Autodesk Inventor part; units mm, degrees
ref_plane "YZ Plane" through (0, 0, 0) normal (1, 0, 0) x (0, 1, 0)
ref_plane "XZ Plane" through (0, 0, 0) normal (0, 1, 0) x (-1, 0, 0)
ref_plane "XY Plane" through (0, 0, 0) normal (0, 0, 1) x (1, 0, 0)
sketch "Sketch1" plane through (0, 0, 0) normal (0, 1, 0) x (-1, 0, 0)
  line L0 (-22.5, 32.5) -> (22.5, 32.5) construction
  line L1 (22.5, 32.5) -> (22.5, -32.5) construction
  line L2 (22.5, -32.5) -> (-22.5, -32.5) construction
  line L3 (-22.5, -32.5) -> (-22.5, 32.5) construction
  line L4 (-22.5, 32.5) -> (22.5, -32.5) construction
  line L5 (22.5, 32.5) -> (-22.5, -32.5) construction
  circle A0 centre (22.5, 32.5) radius 1.5
  circle A1 centre (22.5, -32.5) radius 1.5
  circle A2 centre (-22.5, -32.5) radius 1.5
  circle A3 centre (-22.5, 32.5) radius 1.5
  line L6 (27.5, 30) -> (-27.5, 30)
  line L7 (-27.5, 30) -> (-27.5, 37.5)
  line L8 (-27.5, 37.5) -> (27.5, 37.5)
  line L9 (27.5, 37.5) -> (27.5, 30)
  line L10 (27.5, -30) -> (27.5, -37.5)
  line L11 (27.5, -37.5) -> (-27.5, -37.5)
  line L12 (-27.5, -37.5) -> (-27.5, -30)
  line L13 (-27.5, -30) -> (27.5, -30)
  circle A4 centre (22.5, 32.5) radius 5
  circle A5 centre (22.5, -32.5) radius 5
  circle A6 centre (-22.5, -32.5) radius 5
  circle A7 centre (-22.5, 32.5) radius 5
  line L14 (-27.5, 37.5) -> (27.5, 37.5)
  line L15 (27.5, 37.5) -> (27.5, -37.5)
  line L16 (27.5, -37.5) -> (-27.5, -37.5)
  line L17 (-27.5, -37.5) -> (-27.5, 37.5)
  line L18 (-27.5, 37.5) -> (27.5, -37.5) construction
  line L19 (27.5, 37.5) -> (-27.5, -37.5) construction
  line L20 (-32.5, 42.5) -> (32.5, 42.5)
  line L21 (32.5, 42.5) -> (32.5, -42.5)
  line L22 (32.5, -42.5) -> (-32.5, -42.5)
  line L23 (-32.5, -42.5) -> (-32.5, 42.5)
  line L24 (-32.5, 42.5) -> (32.5, -42.5) construction
  line L25 (32.5, 42.5) -> (-32.5, -42.5) construction
  line L26 (32.5, 42.5) -> (-14.872, 42.5)
  line L27 (0, 0) -> (0, -184) construction
  line L28 (-21, -47.5) -> (21, -47.5)
  line L29 (21, -47.5) -> (21, -89.5)
  line L30 (21, -89.5) -> (-21, -89.5)
  line L31 (-21, -89.5) -> (-21, -47.5)
  line L32 (-21, -47.5) -> (21, -89.5) construction
  line L33 (21, -47.5) -> (-21, -89.5) construction
  line L34 (32.5, -42.5) -> (32.5, -94.5)
  line L35 (32.5, -94.5) -> (-32.5, -94.5)
  line L36 (-32.5, -94.5) -> (-32.5, -42.5)
  line L37 (22.5, 27.5) -> (27.5, 27.5)
  line L38 (22.5, -27.5) -> (27.5, -27.5)
  line L39 (-22.5, -27.5) -> (-27.5, -27.5)
  line L40 (-22.5, 27.5) -> (-27.5, 27.5)
  line L41 (0, 0) -> (0, 113) construction
  line L42 (32.5, 42.5) -> (32.5, 97.5)
  line L43 (32.5, 97.5) -> (-32.5, 97.5)
  line L44 (-32.5, 97.5) -> (-32.5, 42.5)
  line L45 (29.5, 42.5) -> (29.5, 97.5)
  line L46 (-29.5, 97.5) -> (-29.5, 42.5)
  line L47 (32.5, 42.5) -> (36.5, 42.5)
  line L48 (36.5, 42.5) -> (36.5, 112.5)
  line L49 (36.5, 112.5) -> (-36.5, 112.5)
  line L50 (-36.5, 112.5) -> (-36.5, 42.5)
  line L51 (-36.5, 42.5) -> (-32.5, 42.5)
  line L52 (-27.5, 37.5) -> (-36.5, 37.5)
  line L53 (-36.5, 37.5) -> (-36.5, 42.5)
  line L54 (-27.5, -27.5) -> (-26.5, -27.5)
  line L55 (-26.5, -27.5) -> (-26.5, 27.5)
  line L56 (0, 112.5) -> (0, 97.5)
  line L57 (-25.05, 112.5) -> (25.05, 112.5)
  line L58 (25.05, 112.5) -> (25.05, 97.5)
  line L59 (25.05, 97.5) -> (-25.05, 97.5)
  line L60 (-25.05, 97.5) -> (-25.05, 112.5)
  line L61 (-25.05, 112.5) -> (25.05, 97.5) construction
  line L62 (25.05, 112.5) -> (-25.05, 97.5) construction
  line L63 (25.05, 109.5) -> (-25.05, 109.5)
  line L64 (36.5, 112.5) -> (-36.5, 112.5)
  line L65 (-36.5, 112.5) -> (-36.5, 116.5)
  line L66 (-36.5, 116.5) -> (36.5, 116.5)
  line L67 (36.5, 116.5) -> (36.5, 112.5)
  line L68 (36.5, 42.5) -> (36.5, 37.5)
  line L69 (36.5, 37.5) -> (32.5, 37.5)
  point P0 (0, -68.5)
  point P1 (18.1699, 30)
  point P2 (18.1699, -30)
  point P3 (-18.1699, -30)
  point P4 (-18.1699, 30)
  point P5 (-32.5, 70)
  point P6 (32.5, 0)
  point P7 (-32.5, 37.5)
  point P8 (0, 105)
  point P9 (-25.05, 97.5)
  dimension "d8" = 10
  dimension "d9" = 10
  dimension "d10" = 10
  dimension "d11" = 10
  dimension "d0" = 45
  dimension "d1" = 65
  dimension "d2" = 3
  dimension "d3" = 3
  dimension "d4" = 3
  dimension "d5" = 3
  dimension "d6" = 2.5
  dimension "d7" = 2.5
  dimension "d12" = 5
  dimension "d13" = 5
  dimension "d17" = 42
  dimension "d18" = 42
  dimension "d19" = 5
  dimension "d20" = 5
  dimension "d38" = 55
  dimension "d39" = 3
  dimension "d40" = 3
  dimension "d41" = 4
  dimension "d42" = 4
  dimension "d43" = 15
  dimension "d57" = 1
  dimension "d72" = 50.1
  dimension "d84" = 7
  dimension "d85" = 3
extrude "Extrusion1" add sketch "Sketch1" along normal blind 6 contours L15 L37 A4 L6 | L6 A4 L9 | L23 L20 L21 L22 | L52 L53 L51 L23 | A4 L6 | L6 A4 | A4 L8 L9 | L6 A7 L8 A4 | L15 L13 A5 L38 | A7 L6 | L6 A7 | A7 L7 L8 | L10 A5 L13 | A5 L13 | A7 L40 L17 L6 | L6 L7 A7 | A5 L13 | L10 L11 A5 | A5 L11 A6 L13 | A6 L13 | L13 A6 | L39 A6 L13 L17 | L22 L34 L35 L36 | L44 L43 L46 L20 | L51 L50 L49 L60 L43 L44 | L11 L12 A6 | A6 L12 L13 | L21 L47 L68 L69 | L65 L66 L67 L49 | L20 L45 L43 L42 | L42 L43 L58 L49 L48 L47 | L49 L56 L63 L60 | L49 L58 L63 L56 | L28 L29 L30 L31
sketch "Sketch3" plane through (0, 6, 0) normal (0, 1, 0) x (1, 0, 0)
  line L0 (-29.5, -97.5) -> (-29.5, -42.5)
  line L1 (-29.5, -42.5) -> (29.5, -42.5)
  circle A0 centre (-22.5, -32.5) radius 1.5
  circle A1 centre (22.5, 32.5) radius 1.5
  circle A2 centre (22.5, -32.5) radius 1.5
  circle A3 centre (-22.5, 32.5) radius 1.5
  arc A4 (-18.1699, -30) -> (-22.5, -27.5) centre (-22.5, -32.5) ccw
  line L2 (-22.5, -27.5) -> (-27.5, -27.5)
  line L3 (-27.5, -27.5) -> (-27.5, 27.5)
  line L4 (-27.5, 27.5) -> (-22.5, 27.5)
  arc A5 (-22.5, 27.5) -> (-18.1699, 30) centre (-22.5, 32.5) ccw
  line L5 (-18.1699, 30) -> (18.1699, 30)
  arc A6 (18.1699, 30) -> (22.5, 27.5) centre (22.5, 32.5) ccw
  line L6 (22.5, 27.5) -> (27.5, 27.5)
  line L7 (27.5, 27.5) -> (27.5, -27.5)
  line L8 (27.5, -27.5) -> (22.5, -27.5)
  arc A7 (22.5, -27.5) -> (18.1699, -30) centre (22.5, -32.5) ccw
  line L9 (18.1699, -30) -> (-18.1699, -30)
  line L10 (32.5, -37.5) -> (32.5, 94.5)
  line L11 (32.5, 94.5) -> (-32.5, 94.5)
  line L12 (-32.5, 94.5) -> (-32.5, -37.5)
  line L13 (-29.5, -97.5) -> (-32.5, -97.5)
  line L14 (-29.5, -97.5) -> (-29.5, -42.5)
  line L15 (-29.5, -42.5) -> (-32.5, -42.5)
  line L16 (-32.5, -42.5) -> (-32.5, -97.5)
  line L17 (29.5, -97.5) -> (32.5, -97.5)
  line L18 (32.5, -97.5) -> (32.5, -42.5)
  line L19 (32.5, -42.5) -> (29.5, -42.5)
  line L20 (-32.5, 0) -> (-27.5, 0)
  line L21 (-27.5, 27.5) -> (-27.5, 94.5)
  line L22 (27.5, 27.5) -> (27.5, 94.5)
  line L23 (32.5, 94.5) -> (-32.5, 94.5)
  line L24 (36.5, -37.5) -> (32.5, -37.5)
  line L25 (27.5, -27.5) -> (27.5, -42.5)
  line L26 (32.5, -31.5) -> (27.5, -31.5)
  line L27 (32.5, -2.5) -> (27.5, -2.5)
  line L28 (27.5, -31.5) -> (27.5, -2.5)
  line L29 (27.5, -17) -> (32.5, -17) construction
  line L30 (-25.05, -97.5) -> (-29.5, -97.5)
  line L31 (-36.5, -116.5) -> (36.5, -116.5)
  line L32 (36.5, -116.5) -> (36.5, -37.5)
  line L33 (-32.5, -37.5) -> (-36.5, -37.5)
  line L34 (-36.5, -37.5) -> (-36.5, -116.5)
  line L35 (29.5, -42.5) -> (29.5, -97.5)
  line L36 (29.5, -97.5) -> (25.05, -97.5)
  line L37 (25.05, -97.5) -> (25.05, -109.5)
  line L38 (25.05, -109.5) -> (-25.05, -109.5)
  line L39 (-25.05, -109.5) -> (-25.05, -97.5)
  line L40 (-27.5, -27.5) -> (-27.5, -42.5)
  line L41 (27.5, 89.5) -> (-27.5, 89.5)
  point P0 (0, 0)
  point P1 (27.5, 0)
  point P2 (30, -2.5)
  point P3 (30, -31.5)
  point P4 (-32.5, -42.5)
  dimension "d44" = 3
  dimension "d45" = 3
  dimension "d48" = 29
  dimension "d49" = 1
  dimension "d107" = 5
extrude "Extrusion3" add sketch "Sketch3" along normal blind 45 contours L13 L16 L15 L0 | L30 L39 L38 L37 L36 L17 L18 L19 L1 L25 L26 L10 L24 L32 L31 L34 L33 L12 L20 L3 L40 L15 L16 L13 | L19 L18 L17 L35 | L25 L7 L27 L10 L26 | L20 L12 L11 L21 L3 | L7 L22 L11 L10 L27 | L21 L11 L22 L41
sketch "Sketch7" plane through (25.05, 0, 109.5) normal (0, 0, -1) x (-1, 0, 0)
  line L0 (4.05, 6) -> (46.05, 6)
  line L1 (0, 0) -> (50.1, 0)
  line L2 (50.1, 0) -> (50.1, 51)
  line L3 (0, 0) -> (0, 51)
  line L4 (25.05, 51) -> (25.05, 0) construction
  line L5 (5.05, 46) -> (45.05, 46)
  line L6 (45.05, 46) -> (45.05, 6)
  line L7 (45.05, 6) -> (5.05, 6)
  line L8 (5.05, 6) -> (5.05, 46)
  line L9 (5.05, 46) -> (45.05, 6) construction
  line L10 (45.05, 46) -> (5.05, 6) construction
  circle A0 centre (45.05, 6) radius 2
  circle A1 centre (45.05, 46) radius 2
  circle A2 centre (5.05, 46) radius 2
  circle A3 centre (5.05, 6) radius 2
  circle A4 centre (25.05, 26) radius 25
  line L11 (0, 51) -> (50.1, 51)
  dimension "d74" = 40
  dimension "d75" = 40
  dimension "d77" = 4
  dimension "d78" = 4
  dimension "d79" = 4
  dimension "d80" = 4
  dimension "d81" = 50
  dimension "d86" = 6
extrude "Extrusion9" cut sketch "Sketch7" against normal blind 45 contours A4 L8 L5 L6 L0 | L0 A4 | A4 L8 | L6 A4 | A4 L5
extrude "Extrusion10" cut sketch "Sketch7" against normal blind 5 contours L8 A3 L0 | L0 A3 L8 | A0 L6 L0 | L0 L6 A0 | A2 L5 L8 | L8 L5 A2 | A1 L5 L6 | L6 L5 A1
sketch "Sketch8" plane through (0, 51, 0) normal (0, 1, 0) x (1, 0, 0)
  line L0 (32.5, 94.5) -> (-32.5, 94.5)
  line L1 (-32.5, 94.5) -> (-32.5, -37.5)
  line L2 (-36.5, -116.5) -> (0, -116.5)
  line L3 (36.5, -116.5) -> (36.5, -37.5)
  line L4 (36.5, -37.5) -> (32.5, -37.5)
  line L5 (32.5, -37.5) -> (32.5, 94.5)
  line L6 (-36.5, -42.5) -> (36.5, -42.5)
  line L7 (-32.5, -37.5) -> (-36.5, -37.5)
  line L8 (-36.5, -37.5) -> (-36.5, -116.5)
  line L9 (0, -109.5) -> (0, -116.5)
  line L10 (0, -116.5) -> (36.5, -116.5)
  line L11 (27.5, -42.5) -> (29.5, -42.5)
  line L12 (29.5, -42.5) -> (29.5, -97.5)
  line L13 (29.5, -97.5) -> (25.05, -97.5)
  line L14 (25.05, -97.5) -> (25.05, -109.5)
  line L15 (25.05, -109.5) -> (0, -109.5)
  line L16 (0, -109.5) -> (-25.05, -109.5)
  line L17 (-25.05, -109.5) -> (-25.05, -97.5)
  line L18 (-25.05, -97.5) -> (-29.5, -97.5)
  line L19 (-29.5, -97.5) -> (-29.5, -42.5)
  line L20 (27.5, 89.5) -> (27.5, -42.5)
  line L21 (-29.5, -42.5) -> (-27.5, -42.5)
  line L22 (-27.5, -42.5) -> (-27.5, 89.5)
  line L23 (-27.5, 89.5) -> (27.5, 89.5)
  point P0 (0, 0)
extrude "Extrusion11" add sketch "Sketch8" along normal blind 4 contours L5 L4 L3 L6 L20 L23 L22 L8 L7 L1 L0 | L3 L10 L9 L15 L14 L13 L12 L6 | L6 L19 L18 L17 L16 L9 L2 L8
properties part number "New_base_v2"
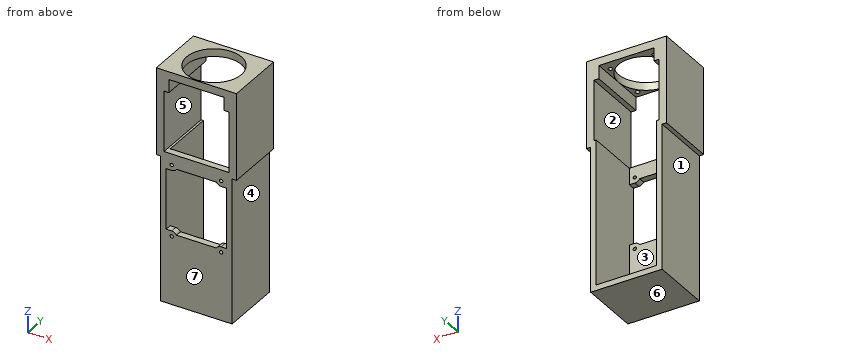
Work out the finished part from the listing and answer in its coordinate system (mm). Face numbers are marked on the shaded views. A direction names the side the tool comes from. Round coordinates to 2 decimals unless told otherwise and drop trailing zeros. Write each loop counter-clockwise with the first axis right and the second up, starting at its lowest first coordinate (ties: lowest second). Pieces come first, ordered by that corner, then holes.
1) A cutting plane is placed at B-B on x = 0. Determine the outline of the cut face in (y, z).
2) Consider probe 1 along X at (y, z) = (35.5, -79.5); probe 2 along Z at (x, y) = (-22.5, 2.6); probe 3 along X at (y, z) = (26, 111). Determine where each line is inside the solid, lowest interval first.
3) Flat-ended cylindrical pins translate along their axes: P1, Ø5, axis at y = 14.5, z = 32, coming from the -X side; P2, Ø16.5, axis at x = -7.5, y = 39, coming from the +Z side; P3, Ø4.5, axis at x = 35, y = 39, coming from the -Z side. Find the tip coordinate at first contact, or state that the pin passes through.
4) Which of the six approach directions +Z, -Z, +X, -X, +Y, -Y give full straight-line access (tool end or side, diameter ignored) to the marked faces 1, 2, 3 and 4?
5) Determine the mould class of the marked faces 5, 6 and 7 for opening direction Z: pulls with the +Z half, pulls with the -Z half, needs draft (parallel to the pull), parting line crosses it, or undercut.
6) A cutting plane is placed at D-D on x = -10. Determine the outline of the cut face in (y, z).
7) A cutting plane is placed at A-A on z = 77.5. Determine the outline of the cut face in (x, y), and give its area (3 significant figures).
Entries:
1. outline: (0, -94.5) - (55, -94.5) - (55, -89.5) - (6, -89.5) - (6, -30) - (0, -30) - close; (0, 30) - (6, 30) - (6, 42.5) - (0, 42.5) - close; (0, 109.5) - (1, 109.5) - (1, 116.5) - (0, 116.5) - close; (51, 109.5) - (55, 109.5) - (55, 116.5) - (51, 116.5) - close
2. probe 1: x = -32.5 to -27.5, 27.5 to 32.5
2. probe 2: z = -94.5 to -34, -31 to -27.5, 27.5 to 31, 34 to 42.5, 109.5 to 116.5
2. probe 3: x = -36.5 to -25, 25 to 36.5
3. P1: stops at x = -32.5
3. P2: stops at z = -89.5
3. P3: stops at z = 37.5
4. face 1: -Z, -X, +Y, -Y
4. face 2: +Y, -Y
4. face 3: +Y
4. face 4: -Z, +X, +Y, -Y
5. face 5: undercut
5. face 6: pulls with the -Z half
5. face 7: needs draft
6. outline: (0, -94.5) - (55, -94.5) - (55, -89.5) - (6, -89.5) - (6, -30) - (0, -30) - close; (0, 30) - (6, 30) - (6, 42.5) - (0, 42.5) - close; (0, 109.5) - (3.09, 109.5) - (3.09, 116.5) - (0, 116.5) - close; (48.91, 109.5) - (55, 109.5) - (55, 116.5) - (48.91, 116.5) - close
7. outline: (-36.5, 0) - (-29.5, 0) - (-29.5, 55) - (-36.5, 55) - close; (29.5, 0) - (36.5, 0) - (36.5, 55) - (29.5, 55) - close
7. area: 770 mm2
